from build123d import *

# Parameters (mm, degrees)
SKETCH1_W           = 105
SKETCH1_H           = 69
BOSS_EXTRUDE1_DEPTH = 5
SKETCH2_W           = 86.836
SKETCH2_H           = 57.499
CUT_EXTRUDE1_DEPTH  = 81.210380614
CUT_EXTRUDE2_DEPTH  = 1
SKETCH4_W           = 5
SKETCH4_H           = 2.165
SKETCH4_H_2         = 0.335
CUT_EXTRUDE3_DEPTH  = 1
CUT_EXTRUDE4_DEPTH  = 81.210380614
SKETCH6_W           = 105
SKETCH6_H           = 69
CUT_EXTRUDE5_DEPTH  = 4


with BuildPart() as part:
    # Sketch1 → Boss-Extrude1 (new body)
    with BuildSketch(Plane(origin=(0, 0, 0), x_dir=(1, 0, 0), z_dir=(0, 1, 0))):
        Rectangle(SKETCH1_W, SKETCH1_H)
    extrude(amount=BOSS_EXTRUDE1_DEPTH)

    # Sketch2 → Cut-Extrude1 (cut, through all)
    with BuildSketch(Plane(origin=(17.072113262, 0, 5.103361153), x_dir=(-1, 0, 0), z_dir=(0, -1, 0))):
        with Locations((16.310113262, 4.341361153)):
            Rectangle(SKETCH2_W, SKETCH2_H)
    extrude(amount=-CUT_EXTRUDE1_DEPTH, mode=Mode.SUBTRACT)

    # Sketch3 → Cut-Extrude2 (cut)
    with BuildSketch(Plane(origin=(17.072113262, 0, 5.103361153), x_dir=(-1, 0, 0), z_dir=(0, -1, 0))):
        Polygon((59.822113262, 30.765861153), (54.524773562, 30.765861153), (54.524773562, -16.234138847), (59.822113262, -16.234138847), (65.822113262, -16.234138847), (65.822113262, 30.765861153), align=None)
    extrude(amount=-CUT_EXTRUDE2_DEPTH, mode=Mode.SUBTRACT)

    # Sketch4 → Cut-Extrude3 (cut)
    with BuildSketch(Plane(origin=(17.072113262, 0, 5.103361153), x_dir=(-1, 0, 0), z_dir=(0, -1, 0))):
        Polygon((-1.187888405, 35.255861153), (3.812111595, 35.255861153), (3.812111595, 33.090861153), (4.312111595, 33.090861153), (4.312111595, 35.755861153), (-1.687888405, 35.755861153), (-1.687888405, 33.090861153), (-1.187888405, 33.090861153), align=None)
        with Locations((1.312111595, 34.173361153)):
            Rectangle(SKETCH4_W, SKETCH4_H)
        Polygon((4.312111595, 33.090861153), (3.812111595, 33.090861153), (3.812111595, 32.755861153), (-1.187888405, 32.755861153), (-1.187888405, 33.090861153), (-1.687888405, 33.090861153), (-1.687888405, 32.255861153), (4.312111595, 32.255861153), align=None)
        with Locations((1.312111595, 32.923361153)):
            Rectangle(SKETCH4_W, SKETCH4_H_2)
    extrude(amount=-CUT_EXTRUDE3_DEPTH, mode=Mode.SUBTRACT)

    # Sketch5 → Cut-Extrude4 (cut, through all)
    with BuildSketch(Plane(origin=(17.072113262, 0, 5.103361153), x_dir=(-1, 0, 0), z_dir=(0, -1, 0))):
        with BuildLine():
            Line((-31.677886738, -0.896638847), (-31.677886738, 11.103361153))
            ThreePointArc((-31.677886738, 11.103361153), (-31.220399504, 12.207833039), (-30.115927617, 12.665320274))
            Line((-30.115927617, 12.665320274), (-28.350143546, 12.665320274))
            ThreePointArc((-28.350143546, 12.665320274), (-27.521232808, 13.008666344), (-27.177886738, 13.837577082))
            Line((-27.177886738, 13.837577082), (-18.865935491, 13.837577082))
            Line((-18.865935491, 13.837577082), (-18.865935491, -4.56597095))
            Line((-18.865935491, -4.56597095), (-27.177886738, -4.56597095))
            ThreePointArc((-27.177886738, -4.56597095), (-27.60841615, -3.526581006), (-28.647806094, -3.096051594))
            Line((-28.647806094, -3.096051594), (-29.478473991, -3.096051594))
            ThreePointArc((-29.478473991, -3.096051594), (-31.033693659, -2.451858515), (-31.677886738, -0.896638847))
        make_face()
    extrude(amount=-CUT_EXTRUDE4_DEPTH, mode=Mode.SUBTRACT)

    # Sketch6 → Cut-Extrude5 (cut)
    with BuildSketch(Plane(origin=(0, 5, 0), x_dir=(1, 0, 0), z_dir=(0, 1, 0))):
        Rectangle(SKETCH6_W, SKETCH6_H)
    extrude(amount=-CUT_EXTRUDE5_DEPTH, mode=Mode.SUBTRACT)


solid = part.part
Here's how the part is built. I have some questions about the finished solid (model axes, mm). Coordinates: 2 decimals unless noted, no trailing zeros. Write each loop counter-clockwise with the first axis right and the second up, starting at its lowest first coordinate (ties: lowest second). Pieces come first, ordered by that corner, then holes.
Item 1: I want a section at C-C on y = 0.2. Write out the boundary of the cut face in (x, z).
Item 2: If I drill on line 1 (X direction, y = 0.7, z = 26); line 2 (Z direction, x = 8.5, y = 0.2); line 3 (Z direction, x = 18, y = 0.3), over which ranges is the centre line in solid material (lowest first)?
Item 3: I want a section at B-B on x = 16. Write out the boundary of the cut face in (y, z).
Item 4: If we mould it in two halves opening along Z, with no side actions, what happens to faces 1 (the flat face through (-0.2, 0, -28.3)), 2 (the cylindrical face through (48.09, 0.49, 7.57))? For each: +Z half, -Z half, draft (parallel to the pull), parting line (faces both ways), or undercut.
Item 5: Will this pin go through, and if not, where does the flat tip stop? pin 1 (8 mm diameter, centred on x = -27, z = 22.5, fed in from -Y).
Item 6: I want a section at A-A on z = 2.5. Write out the boundary of the cut face in (x, y).
Findings below:
1. outline: (-52.5, -34.5) - (52.5, -34.5) - (52.5, 34.5) - (-52.5, 34.5) - close; hole (-48.75, -25.66) - (-42.66, -25.66) - (-42.66, -27.99) - (12.76, -27.99) - (12.76, -30.65) - (18.76, -30.65) - (18.76, -27.99) - (44.18, -27.99) - (44.18, -8.73) - (44.25, -8.73) arc R1.17 cw to (45.42, -7.56) - (47.19, -7.56) arc R1.56 ccw to (48.75, -6) - (48.75, 6) arc R2.2 ccw to (46.55, 8.2) - (45.72, 8.2) arc R1.47 cw to (44.25, 9.67) - (44.18, 9.67) - (44.18, 29.51) - (-42.66, 29.51) - (-42.66, 21.34) - (-48.75, 21.34) - close
2. line 1: x = -52.5 to -42.66, 44.18 to 52.5
2. line 2: z = -34.5 to -27.99, 29.51 to 34.5
2. line 3: z = -34.5 to -30.65, 29.51 to 34.5
3. outline: (0, -34.5) - (1, -34.5) - (1, -30.65) - (0, -30.65) - close; (0, 29.51) - (1, 29.51) - (1, 34.5) - (0, 34.5) - close
4. face 1: draft
4. face 2: undercut
5. pin 1: passes through
6. outline: (-52.5, 0) - (-48.75, 0) - (-48.75, 1) - (-52.5, 1) - close; (48.75, 0) - (52.5, 0) - (52.5, 1) - (48.75, 1) - close
